```python
from build123d import *

# Parameters (mm, degrees)
CYLINDER003_W     = 6.4
CYLINDER003_H     = 22
CYLINDER003_ANGLE = 90
BOX004_W          = 10
BOX004_H          = 12.1
BOX004_DEPTH      = 22
CYLINDER002_W     = 6.4
CYLINDER002_H     = 22
CYLINDER002_ANGLE = 90
BOX003_W          = 10
BOX003_H          = 12.1
BOX003_DEPTH      = 22
BOX002_W          = 2
BOX002_H          = 11
BOX002_DEPTH      = 22
CYLINDER001_R     = 1.75
CYLINDER001_DEPTH = 18
CYLINDER_R        = 4.15
CYLINDER_DEPTH    = 22
BOX001_W          = 13
BOX001_H          = 21
BOX001_DEPTH      = 10


with BuildPart() as cylinder003:
    # Cylinder003 → Cylinder003 (revolve)
    with BuildSketch(Plane(origin=(25, -6.85, -3), x_dir=(-1, 0, 0), z_dir=(0, 1, 0))):
        with Locations((3.2, 11)):
            Rectangle(CYLINDER003_W, CYLINDER003_H)
    revolve(axis=Axis((25, -6.85, -3), (0, 0, 1)), revolution_arc=CYLINDER003_ANGLE)


with BuildPart() as cut004:
    # Box004 → Box004 (new body)
    with BuildSketch(Plane(origin=(11.5, -19, -3), x_dir=(1, 0, 0), z_dir=(0, 0, 1))):
        with Locations((5, 6.05)):
            Rectangle(BOX004_W, BOX004_H)
    extrude(amount=BOX004_DEPTH)

    # Cut004: cut Cylinder003
    add(cylinder003.part, mode=Mode.SUBTRACT)


with BuildPart() as cylinder002:
    # Cylinder002 → Cylinder002 (revolve)
    with BuildSketch(Plane(origin=(25, -6.85, -3), x_dir=(0, -1, 0), z_dir=(-1, 0, 0))):
        with Locations((3.2, 11)):
            Rectangle(CYLINDER002_W, CYLINDER002_H)
    revolve(axis=Axis((25, -6.85, -3), (0, 0, 1)), revolution_arc=CYLINDER002_ANGLE)


with BuildPart() as cut003:
    # Box003 → Box003 (new body)
    with BuildSketch(Plane(origin=(28.5, -19, -3), x_dir=(1, 0, 0), z_dir=(0, 0, 1))):
        with Locations((5, 6.05)):
            Rectangle(BOX003_W, BOX003_H)
    extrude(amount=BOX003_DEPTH)

    # Cut003: cut Cylinder002
    add(cylinder002.part, mode=Mode.SUBTRACT)


with BuildPart() as cube002:
    # Box002 → Box002 (new body)
    with BuildSketch(Plane(origin=(24, -21, -3), x_dir=(1, 0, 0), z_dir=(0, 0, 1))):
        with Locations((1, 5.5)):
            Rectangle(BOX002_W, BOX002_H)
    extrude(amount=BOX002_DEPTH)


with BuildPart() as cylinder001:
    # Cylinder001 → Cylinder001 (new body)
    with BuildSketch(Plane(origin=(16, -15, 5), x_dir=(0, 0, -1), z_dir=(1, 0, 0))):
        Circle(CYLINDER001_R)
    extrude(amount=CYLINDER001_DEPTH)


with BuildPart() as cylinder:
    # Cylinder → Cylinder (new body)
    with BuildSketch(Plane(origin=(25, -6.85, -3), x_dir=(1, 0, 0), z_dir=(0, 0, 1))):
        Circle(CYLINDER_R)
    extrude(amount=CYLINDER_DEPTH)


with BuildPart() as cut006:
    # Box001 → Box001 (new body)
    with BuildSketch(Plane(origin=(18.5, -19, 0), x_dir=(1, 0, 0), z_dir=(0, 0, 1))):
        with Locations((6.5, 10.5)):
            Rectangle(BOX001_W, BOX001_H)
    extrude(amount=BOX001_DEPTH)

    # Cut: cut Cylinder
    add(cylinder.part, mode=Mode.SUBTRACT)

    # Cut001: cut Cylinder001
    add(cylinder001.part, mode=Mode.SUBTRACT)

    # Cut002: cut Cube002
    add(cube002.part, mode=Mode.SUBTRACT)

    # Cut005: cut Cut003
    add(cut003.part, mode=Mode.SUBTRACT)

    # Cut006: cut Cut004
    add(cut004.part, mode=Mode.SUBTRACT)


with BuildPart() as cut006_1:
    # Cut006 placement: moved
    add(cut006.part.moved(Location((0, -2, 12))))


solid = cut006_1.part
```
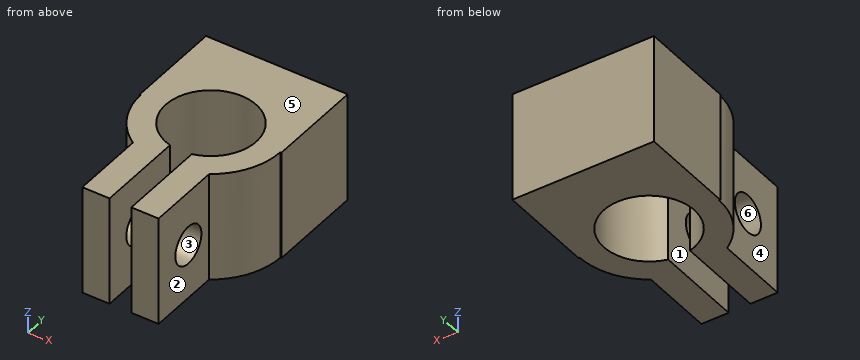
Model file for the job. Use its own axes, mm. Face numbers are marked on the shaded views. A direction names the side the tool comes from. Give positions to 0.01 mm unless a question says otherwise; leave off trailing zeros. Write each loop counter-clockwise with the first axis right and the second up, starting at its lowest first coordinate (ties: lowest second). Pieces come first, ordered by that corner, then holes. Notation, with made-up numbers: M -12.5,42 L 30.5,42 A26 cw 30.5,68 Z; hole C 0.25,-28 d1. An arc over 180 degrees is marked long. Use a Markdown table: item, result.
1) Drill centre lines: line 1 (X direction, y = -15.5, z = 12.75); line 2 (X direction, y = -8.85, z = 18); line 3 (Y direction, x = 23.4, z = 17). Where is each one in solid material? Low to high. Write a range as from..to.
Responses:
| item | result |
|---|---|
| line 1 | x = 21.5..24, 26..28.5 |
| line 2 | x = 18.5..20.85, 29.15..31.5 |
| line 3 | y = -21..-18.75, -15.25..-12.68, -5.02..0 |
2) Cut at C-C (x = 22). List the corners of the cut face in (y, z), and give its area (3 significant figures).
Responses:
| item | result |
|---|---|
| outline | M -21,12 L -11.72,12 L -11.72,22 L -21,22 Z; M -5.98,12 L 0,12 L 0,22 L -5.98,22 Z; hole C -17,17 d3.5 |
| area | 143 mm2 |
3) Pull direction Z, two halves, no side cores. Call the marked faces 4, 5 and 6: +Z half, -Z half, draft (parallel to the pull), parting line (faces both ways), or undercut.
Responses:
| item | result |
|---|---|
| face 4 | draft |
| face 5 | +Z half |
| face 6 | undercut |
4) Pin check, flat tips, straight feed: pin 1 (3.5 mm diameter, centred on y = -18.5, z = 19.5, fed in from -X); pin 2 (1 mm diameter, centred on x = 29.5, z = 19.5, fed in from +Y); pin 3 (3 mm diameter, centred on y = -10.5, z = 20.5, fed in from -X); pin 4 (2.5 mm diameter, centred on y = -16, z = 17.5, fed in from +X). Stop position of each tip, or through.
Responses:
| item | result |
|---|---|
| pin 1 | stops at x = 21.5 |
| pin 2 | stops at y = 0 |
| pin 3 | stops at x = 18.6 |
| pin 4 | stops at x = 28.5 |
5) Cut at A-A (z = 17). List the corners of the cut face in (x, y), and give its area (3 significant figures).
Responses:
| item | result |
|---|---|
| outline | M 18.5,-8.9 L 18.6,-8.9 A6.4 ccw 21.5,-14.21 L 21.5,-15.25 L 24,-15.25 L 24,-12.88 A4.15 cw long 26,-12.88 L 26,-15.25 L 28.5,-15.25 L 28.5,-14.21 A6.4 ccw 31.4,-8.9 L 31.5,-8.9 L 31.5,0 L 18.5,0 Z; M 21.5,-21 L 24,-21 L 24,-18.75 L 21.5,-18.75 Z; M 26,-21 L 28.5,-21 L 28.5,-18.75 L 26,-18.75 Z |
| area | 134 mm2 |
6) Tool access for the marked faces 1, 2 and 3: list every direction of +Z, -Z, +X, -X, +Y, -Y with a clear straight run to the whole face (end or side of a thin tool).
Responses:
| item | result |
|---|---|
| face 1 | +Z, -Z, -Y |
| face 2 | +Z, -Z, +X, -Y |
| face 3 | +X, -X |
7) Cut at D-D (z = 13). List the corners of the cut face in (x, y), and give its area (3 significant figures).
Responses:
| item | result |
|---|---|
| outline | M 18.5,-8.9 L 18.6,-8.9 A6.4 ccw 21.5,-14.21 L 21.5,-21 L 24,-21 L 24,-12.88 A4.15 cw long 26,-12.88 L 26,-21 L 28.5,-21 L 28.5,-14.21 A6.4 ccw 31.4,-8.9 L 31.5,-8.9 L 31.5,0 L 18.5,0 Z |
| area | 152 mm2 |
8) Cut at B-B (y = -12). List the corners of the cut face in (x, z), and give its area (3 significant figures).
Responses:
| item | result |
|---|---|
| outline | M 19.43,12 L 22.3,12 L 22.3,22 L 19.43,22 Z; M 27.7,12 L 30.57,12 L 30.57,22 L 27.7,22 Z |
| area | 57.4 mm2 |
